Build history of the part. All positions in model axes, mm. A direction names the side the tool comes from. Coordinates: 2 decimals unless noted, no trailing zeros. Loops run counter-clockwise (first coordinate to the right, second up) from the corner with the lowest first, then second, coordinate; pieces in that order, holes last.
Item 1: Cut at A-A (y = -10.5). List the corners of the cut face in (x, z).
Item 2: Flat gauge pins, fed straight in: pin 1 (2 mm diameter, centred on y = -10, z = -3.5, fed in from -X); pin 2 (10.5 mm diameter, centred on x = 0.5, y = 5.5, fed in from -Z); pin 3 (0.5 mm diameter, centred on y = 15, z = -1, fed in from -X); pin 4 (2 mm diameter, centred on x = 8.5, z = -0.5, fed in from +Y). Where does each tip first touch, or does it go through?
Item 3: Mould opens along X. For faces 3 (the face through (7.002, -12.913, -1.588)), 4 (the face through (6.5, 13, -1)), 5 (the face through (1, 0, 1)), 6 (the face through (11, 13, -3)) say: released by +X, released by -X, zero draft, split by the parting line, or undercut.
Item 4: 3-axis set-ups, long thin cutter, end or side, ignore diameter. For faces 1 (the face through (3.1, -19, 0.2)), 2 (the face through (0, 0, 0)): which of +Z, -Z, +X, -X, +Y, -Y reach the whole face in a straight line?
Item 5: Drill centre lines: line 1 along Y through (x, z) = (-1, 0.7); line 2 along Y through (x, z) = (10.5, -2.95); line 3 along X through (y, z) = (-10.5, -1.5). Where is each one in solid material? Low to high.
Item 6: Cut at B-B (x = -1). List the corners of the cut face in (y, z), and give its area (3 significant figures).
Item 7: Cut at D-D (y = -16). List the corners of the cut face in (x, z).
Item 8: Cut at C-C (z = -0.8). List the corners of the cut face in (x, y).
from build123d import *

# Parameters (mm, degrees)
SKETCH_1_W          = 13
SKETCH_1_H          = 38
EXTRUDE_1_DEPTH     = 1
SKETCH_2_R          = 2
EXTRUDE_2_DEPTH     = 38
CUT_EXTRUDE_1_DEPTH = 10
SKETCH_4_R          = 2.5
CUT_EXTRUDE_2_DEPTH = 2


with BuildPart() as part:
    # 草图1 → 凸台-拉伸1 (new body)
    with BuildSketch(Plane.XY):
        Rectangle(SKETCH_1_W, SKETCH_1_H)
    extrude(amount=EXTRUDE_1_DEPTH)

    # 草图2 → 凸台-拉伸2 (add)
    with BuildSketch(Plane(origin=(0, 19, 0), x_dir=(1, 0, 0), z_dir=(0, 1, 0))):
        with BuildLine():
            Line((6.5, -1), (9, -1))
            ThreePointArc((9, -1), (10.767766953, 3.267766953), (6.5, 1.5))
            Line((6.5, 1.5), (6.5, -1))
        make_face()
        with Locations((9, 1.5)):
            Circle(SKETCH_2_R, mode=Mode.SUBTRACT)
    extrude(amount=-EXTRUDE_2_DEPTH)

    # 草图3 → 切除-拉伸1 (cut)
    with BuildSketch(Plane.XY.offset(1)):
        Polygon((5.519068854, -7.009502005), (12.519042916, -6.99044612), (12.480931146, 7.009502005), (5.480957084, 6.99044612), align=None)
    extrude(amount=-CUT_EXTRUDE_1_DEPTH, mode=Mode.SUBTRACT)

    # 草图4 → 切除-拉伸2 (cut)
    with BuildSketch(Plane(origin=(0, 0, 0), x_dir=(-1, 0, 0), z_dir=(0, 0, -1))):
        with Locations((1, 12.5)):
            Circle(SKETCH_4_R)
        with Locations((1, -12.5)):
            Circle(SKETCH_4_R)
    extrude(amount=-CUT_EXTRUDE_2_DEPTH, mode=Mode.SUBTRACT)


solid = part.part
Filled sheet:
1. outline: (-6.5, 0) - (-2.5, 0) - (-2.5, 1) - (-6.5, 1) - close; (0.5, 0) - (6.5, 0) - (6.5, -1.5) arc R2.5 ccw (long way) to (9, 1) - (0.5, 1) - close; hole circle Ø4 at (9, -1.5)
2. pin 1: stops at x = 6.71
2. pin 2: stops at z = 0
2. pin 3: stops at x = 6.5
2. pin 4: stops at y = 19
3. face 3: undercut
3. face 4: released by -X
3. face 5: zero draft
3. face 6: split by the parting line
4. face 1: +Z, -Z, +X, -X, -Y
4. face 2: -Z, -X, +Y, -Y
5. line 1: y = -19 to -15, -10 to 10, 15 to 19
5. line 2: y = -19 to -7, 7 to 19
5. line 3: x = 6.5 to 7, 11 to 11.5
6. outline: (-19, 0) - (-15, 0) - (-15, 1) - (-19, 1) - close; (-10, 0) - (10, 0) - (10, 1) - (-10, 1) - close; (15, 0) - (19, 0) - (19, 1) - (15, 1) - close
6. area: 28.0 mm2
7. outline: (-6.5, 0) - (6.5, 0) - (6.5, -1.5) arc R2.5 ccw (long way) to (9, 1) - (-6.5, 1) - close; hole circle Ø4 at (9, -1.5)
8. outline: (6.5, -19) - (7.13, -19) - (7.13, -7.01) - (6.5, -7.01) - close; (6.5, 6.99) - (7.13, 6.99) - (7.13, 19) - (6.5, 19) - close; (10.87, -19) - (11.4, -19) - (11.4, -6.99) - (10.87, -6.99) - close; (10.87, 7.01) - (11.4, 7.01) - (11.4, 19) - (10.87, 19) - close
